The listing builds one solid part. Answer for the finished solid, in the listing's coordinates (mm). A direction names the side the tool comes from. Coordinates: 2 decimals unless noted, no trailing zeros. Order: outer loops, then holes, each group sorted by start corner. A loop starts at its lowest first (then second) coordinate and runs counter-clockwise, first axis right, second up. Notation, with made-up numbers: (35.25, 84) -> (67.25, 84) arc R26 ccw to (67.25, 105) -> close; hole circle Ø10 at (21, 84). An arc over 180 degrees is marked (long way). Return JSON: item names as keys, results as strings.
from build123d import *

# Parameters (mm, degrees)
SKETCH_1_W                         = 120
SKETCH_1_H                         = 42
SM_BASE_FLANGE_1_DEPTH             = 3
SM_EDGE_FLANGE_1_STRIP_W           = 13.4732
SM_EDGE_FLANGE_1_STRIP_H           = 3
SM_EDGE_FLANGE_1_STRIP_CUT_DEPTH   = 42
SM_EDGE_FLANGE_1_STRIP_2_W         = 13.4732
SM_EDGE_FLANGE_1_STRIP_2_H         = 3
SM_EDGE_FLANGE_1_STRIP_CUT_2_DEPTH = 42
SM_EDGE_FLANGE_1_DEPTH             = 42
SM_EDGE_FLANGE_1_BEND_DEPTH        = 42
SM_EDGE_FLANGE_2_STRIP_W           = 13.4732
SM_EDGE_FLANGE_2_STRIP_H           = 3
SM_EDGE_FLANGE_2_STRIP_CUT_DEPTH   = 42
SM_EDGE_FLANGE_2_STRIP_2_W         = 13.4732
SM_EDGE_FLANGE_2_STRIP_2_H         = 3
SM_EDGE_FLANGE_2_STRIP_CUT_2_DEPTH = 42
SM_EDGE_FLANGE_2_DEPTH             = 42
SM_EDGE_FLANGE_2_BEND_DEPTH        = 42
FILLET_1_R                         = 5
HOLE_WIZARD_M6_1_D                 = 5
HOLE_WIZARD_M4_1_D                 = 4.5


# Sheet-metal steps are written as plain solids
with BuildPart() as part:
    # Sketch 1 → 베이스-플랜지1 (new body)
    with BuildSketch(Plane(origin=(0, 0, 0), x_dir=(1, 0, 0), z_dir=(0, 1, 0))):
        Rectangle(SKETCH_1_W, SKETCH_1_H)
    extrude(amount=-SM_BASE_FLANGE_1_DEPTH)

    # 모서리 플랜지1 strip (across the edge) → 모서리 플랜지1 strip cut (cut)
    with BuildSketch(Plane(origin=(-60, -3, 21), x_dir=(1, 0, 0), z_dir=(0, 0, -1))):
        with Locations((-3, -1.5)):
            Rectangle(SM_EDGE_FLANGE_1_STRIP_W, SM_EDGE_FLANGE_1_STRIP_H)
    extrude(amount=SM_EDGE_FLANGE_1_STRIP_CUT_DEPTH, mode=Mode.SUBTRACT)

    # 모서리 플랜지1 strip 2 (across the edge) → 모서리 플랜지1 strip cut 2 (cut)
    with BuildSketch(Plane(origin=(60, -3, -21), x_dir=(-1, 0, 0), z_dir=(0, 0, 1))):
        with Locations((-3, -1.5)):
            Rectangle(SM_EDGE_FLANGE_1_STRIP_2_W, SM_EDGE_FLANGE_1_STRIP_2_H)
    extrude(amount=SM_EDGE_FLANGE_1_STRIP_CUT_2_DEPTH, mode=Mode.SUBTRACT)

    # 모서리 플랜지1 section (across the edge) → 모서리 플랜지1 (add)
    with BuildSketch(Plane(origin=(-60, -3, 21), x_dir=(1, 0, 0), z_dir=(0, 0, -1))):
        with BuildLine():
            Line((0, 0.7366), (0, 21))
            Line((0, 21), (3, 21))
            Line((3, 21), (3, 0.7366))
            ThreePointArc((3, 0.7366), (3.215745145, 0.215745145), (3.7366, 0))
            Line((3.7366, 0), (3.7366, -3))
            ThreePointArc((3.7366, -3), (1.094424801, -1.905575199), (0, 0.7366))
        make_face()
    extrude(amount=SM_EDGE_FLANGE_1_DEPTH)

    # 모서리 플랜지1 section 2 (across the edge) → 모서리 플랜지1 bend (add)
    with BuildSketch(Plane(origin=(60, -3, -21), x_dir=(-1, 0, 0), z_dir=(0, 0, 1))):
        with BuildLine():
            Line((0, 0.7366), (0, 21))
            Line((0, 21), (3, 21))
            Line((3, 21), (3, 0.7366))
            ThreePointArc((3, 0.7366), (3.215745145, 0.215745145), (3.7366, 0))
            Line((3.7366, 0), (3.7366, -3))
            ThreePointArc((3.7366, -3), (1.094424801, -1.905575199), (0, 0.7366))
        make_face()
    extrude(amount=SM_EDGE_FLANGE_1_BEND_DEPTH)

    # 모서리 플랜지2 strip (across the edge) → 모서리 플랜지2 strip cut (cut)
    with BuildSketch(Plane(origin=(-60, -24, -21), x_dir=(0, 1, 0), z_dir=(0, 0, 1))):
        with Locations((-3, -1.5)):
            Rectangle(SM_EDGE_FLANGE_2_STRIP_W, SM_EDGE_FLANGE_2_STRIP_H)
    extrude(amount=SM_EDGE_FLANGE_2_STRIP_CUT_DEPTH, mode=Mode.SUBTRACT)

    # 모서리 플랜지2 strip 2 (across the edge) → 모서리 플랜지2 strip cut 2 (cut)
    with BuildSketch(Plane(origin=(60, -24, 21), x_dir=(0, 1, 0), z_dir=(0, 0, -1))):
        with Locations((-3, -1.5)):
            Rectangle(SM_EDGE_FLANGE_2_STRIP_2_W, SM_EDGE_FLANGE_2_STRIP_2_H)
    extrude(amount=SM_EDGE_FLANGE_2_STRIP_CUT_2_DEPTH, mode=Mode.SUBTRACT)

    # 모서리 플랜지2 section (across the edge) → 모서리 플랜지2 (add)
    with BuildSketch(Plane(origin=(-60, -24, -21), x_dir=(0, 1, 0), z_dir=(0, 0, 1))):
        with BuildLine():
            Line((0, 0.7366), (0, 20))
            Line((0, 20), (3, 20))
            Line((3, 20), (3, 0.7366))
            ThreePointArc((3, 0.7366), (3.215745145, 0.215745145), (3.7366, 0))
            Line((3.7366, 0), (3.7366, -3))
            ThreePointArc((3.7366, -3), (1.094424801, -1.905575199), (0, 0.7366))
        make_face()
    extrude(amount=SM_EDGE_FLANGE_2_DEPTH)

    # 모서리 플랜지2 section 2 (across the edge) → 모서리 플랜지2 bend (add)
    with BuildSketch(Plane(origin=(60, -24, 21), x_dir=(0, 1, 0), z_dir=(0, 0, -1))):
        with BuildLine():
            Line((0, 0.7366), (0, 20))
            Line((0, 20), (3, 20))
            Line((3, 20), (3, 0.7366))
            ThreePointArc((3, 0.7366), (3.215745145, 0.215745145), (3.7366, 0))
            Line((3.7366, 0), (3.7366, -3))
            ThreePointArc((3.7366, -3), (1.094424801, -1.905575199), (0, 0.7366))
        make_face()
    extrude(amount=SM_EDGE_FLANGE_2_BEND_DEPTH)

    # 필렛1
    fillet_1_edges = [part.edges().sort_by_distance(p)[0] for p in [
        (-80, -22.5, -21),
        (-80, -22.5, 21),
        (80, -22.5, 21),
        (80, -22.5, -21),
    ]]
    fillet(fillet_1_edges, radius=FILLET_1_R)

    # M6 탭을 위한 탭 드릴1 (through all)
    with Locations(Plane(origin=(0, -24, 0), x_dir=(-1, 0, 0), z_dir=(0, -1, 0))):
        with Locations((-70, 10), (-70, -10), (70, 10), (70, -10)):
            Hole(HOLE_WIZARD_M6_1_D / 2)

    # M4 여유 구멍1 (through all)
    with Locations(Plane(origin=(0, 0, 0), x_dir=(1, 0, 0), z_dir=(0, 1, 0))):
        with Locations((-45, 7), (0, -7), (45, 7)):
            Hole(HOLE_WIZARD_M4_1_D / 2)


solid = part.part
1. Determine the mould class of faces 4 (the face through (79, -22, 19)), 5 (the face through (58.07, -22.88, 0.29)), 6 (the face through (0, -2, -21)) for opening direction X: pulls with the +X half, pulls with the -X half, needs draft (parallel to the pull), parting line crosses it, or undercut.
Answer block:
{"face 4": "pulls with the +X half", "face 5": "undercut", "face 6": "needs draft"}
2. Consider line 1 (X direction, y = -11.5, z = 5); line 2 (X direction, y = -21.95, z = -10); line 3 (Z direction, x = -45, y = -2.05). Determine where each line is inside the solid, lowest interval first. Write a range as from..to.
Answer block:
{"line 1": "x = -60..-57, 57..60", "line 2": "x = -80..-72.5, -67.5..-57.4, 57.4..67.5, 72.5..80", "line 3": "z = -21..-9.25, -4.75..21"}
3. Each of these flat-tipped pins is pushed along its axis until it touches: pin 1 Ø8.5 at (y, z) = (-12.5, 5) entering from +X; pin 2 Ø6 at (x, z) = (-37, -12) entering from -Y; pin 3 Ø4.5 at (x, z) = (70, -10) entering from +Y; pin 4 Ø8.5 at (y, z) = (-16, 0) entering from -X. Where does it stop, or does it pass through?
Answer block:
{"pin 1": "stops at x = 60", "pin 2": "stops at y = -3", "pin 3": "passes through", "pin 4": "stops at x = -60"}
4. The part is cut by section C-C on z = -2.5. Give the vertices of the cut face in (x, y), and give its area (3 significant figures).
Answer block:
{"outline": "(-80, -24) -> (-60.74, -24) arc R3.74 ccw to (-57, -20.26) -> (-57, -3.74) arc R0.74 cw to (-56.26, -3) -> (56.26, -3) arc R0.74 cw to (57, -3.74) -> (57, -20.26) arc R3.74 ccw to (60.74, -24) -> (80, -24) -> (80, -21) -> (60.74, -21) arc R0.74 cw to (60, -20.26) -> (60, -3.74) arc R3.74 ccw to (56.26, 0) -> (-56.26, 0) arc R3.74 ccw to (-60, -3.74) -> (-60, -20.26) arc R0.74 cw to (-60.74, -21) -> (-80, -21) -> close", "area": "594 mm2"}
5. The part is cut by section B-B on x = -45. Give the vertices of the cut face in (y, z).
Answer block:
{"outline": "(-3, -21) -> (0, -21) -> (0, -9.25) -> (-3, -9.25) -> close; (-3, -4.75) -> (0, -4.75) -> (0, 21) -> (-3, 21) -> close"}
6. For faces 1 (the face through (79, -22, -19)), 2 (the face through (-1, -3, 0)), 3 (the face through (71, -21, 0)), determine the directions among +Z, -Z, +X, -X, +Y, -Y from which every point of the face is accessible in a straight line to the end or side of a thin tool.
Answer block:
{"face 1": "-Z, +X, +Y, -Y", "face 2": "+Z, -Z, -Y", "face 3": "+Z, -Z, +X, +Y"}
7. The part is cut by section D-D on x = -29. Give the vertices of the cut face in (y, z), and give its area (3 significant figures).
Answer block:
{"outline": "(-3, -21) -> (0, -21) -> (0, 21) -> (-3, 21) -> close", "area": "126 mm2"}
8. The part is cut by section A-A on y = -12.75. Give the vertices of the cut face in (x, z), and give its area (3 significant figures).
Answer block:
{"outline": "(-60, -21) -> (-57, -21) -> (-57, 21) -> (-60, 21) -> close; (57, -21) -> (60, -21) -> (60, 21) -> (57, 21) -> close", "area": "252 mm2"}
